from build123d import *

# Parameters (mm, degrees)
F1_DEPTH  = 15
F2_R      = 3.5
F3_DEPTH  = 25
F5_D      = 6.6
F5_DEPTH  = 15
F5_TIP    = 1.9828400428
F6_SIZE   = 10
F7_W      = 6.5
F7_H      = 6.5
F8_DEPTH  = 12.8004791855
F10_D     = 4.4
F10_DEPTH = 5
F10_TIP   = 1.3218933619
F11_SIZE  = 0.25
F12_R     = 0.25


with BuildPart() as f1:
    # F0 (on Top) → F1 (new body)
    with BuildSketch(Plane.XY):
        with BuildLine():
            Line((20, -20), (20, 20))
            Line((20, 20), (-20, 20))
            Line((-20, 20), (-20, 1.5))
            Line((-20, 1.5), (-7.7562877719, 1.5))
            ThreePointArc((-7.7562877719, 1.5), (7.9, 0), (-7.7562877719, -1.5))
            Line((-7.7562877719, -1.5), (-20, -1.5))
            Line((-20, -1.5), (-20, -20))
            Line((-20, -20), (20, -20))
        make_face()
    extrude(amount=F1_DEPTH)

    # F2 (on Front) → F3 (cut)
    with BuildSketch(Plane.XZ):
        with Locations((-14, 7.5)):
            Circle(F2_R)
    extrude(amount=F3_DEPTH, mode=Mode.SUBTRACT)

    # F5
    with Locations(Plane.XZ.offset(-1.5)):
        with Locations((-14, 7.5)):
            Hole(F5_D / 2, depth=F5_DEPTH)
            with Locations((0, 0, -(F5_DEPTH + F5_TIP / 2))):  # 118° drill point
                Cone(0, F5_D / 2, F5_TIP, mode=Mode.SUBTRACT)

    # F6
    f6_edges = [f1.edges().sort_by_distance(p)[0] for p in [
        (20, -20, 7.5),
        (20, 20, 7.5),
    ]]
    chamfer(f6_edges, length=F6_SIZE)

    # F7 (on face) → F8 (cut, through all)
    with BuildSketch(Plane.YZ.offset(20)):
        with Locations((0, 7.5)):
            Rectangle(F7_W, F7_H)
    extrude(amount=-F8_DEPTH, mode=Mode.SUBTRACT)

    # F10
    with Locations(Plane(origin=(0, 0, 0), x_dir=(1, 0, 0), z_dir=(0, 0, -1))):
        with Locations((14, 0)):
            Hole(F10_D / 2, depth=F10_DEPTH)
            with Locations((0, 0, -(F10_DEPTH + F10_TIP / 2))):  # 118° drill point
                Cone(0, F10_D / 2, F10_TIP, mode=Mode.SUBTRACT)

    # F11
    f11_edges = [f1.edges().sort_by_distance(p)[0] for p in [
        (-17.5, -20, 7.5),
        (11.8, 0, 0),
    ]]
    chamfer(f11_edges, length=F11_SIZE)

    # F12
    f12_edges = [f1.edges().sort_by_distance(p)[0] for p in [
        (13.60026, 3.25, 4.25),
        (13.60026, -3.25, 4.25),
        (13.60026, 3.25, 10.75),
        (13.60026, -3.25, 10.75),
    ]]
    fillet(f12_edges, radius=F12_R)


solid = f1.part
Check sheet for the modelled part. Datum: model origin and axes. Units: mm. A direction names the side the tool comes from. Round coordinates to 2 decimals unless told otherwise and drop trailing zeros. Loops run counter-clockwise (first coordinate to the right, second up) from the corner with the lowest first, then second, coordinate; pieces in that order, holes last.
1. Gauge pin test, flat ends, axial feed: pin 1 Ø3.5 at (x, y) = (14, 0) entering from -Z; pin 2 Ø6.5 at (x, z) = (15, 6.5) entering from +Y; pin 3 Ø5.5 at (x, z) = (-14, 7.5) entering from -Y. Record the tip position at first contact, or that the pin passes through.
2. Scan lines: probe 1 along Y at (x, z) = (8, 9.5); probe 2 along X at (y, z) = (0, 2.9); probe 3 along Y at (x, z) = (0, 8.75). Record each from-to range of solid material in increasing order.
3. Sectioned sample at A-A on y = 0. Record the boundary of the cut face in (x, z), and give its area (3 significant figures).
4. Sectioned sample at D-D on y = 6. Record the boundary of the cut face in (x, z), and give its area (3 significant figures).
5. Set-up check for faces 1 (the flat face through (14, 0, 10.75)), 2 (the cylindrical face through (-11.381, 9.105, 5.492)), 3 (the cylindrical face through (11.968, 0.843, 2.278)), 4 (the flat face through (-14, 1.5, 4)): record each of +Z, -Z, +X, -X, +Y, -Y from which the full face is reachable in a straight line by a thin tool's end or side.
6. Sectioned sample at C-C on z = 1.75. Record the boundary of the cut face in (x, y).
7. Mould release check, pull along Z, two halves, no side actions. Record for faces 5 (the flat face through (-12, -1.5, 4)), 6 (the cylindrical face through (-10.767, -10.497, 6.159)), 7 (the flat face through (-9, -4, 0)): released by +Z, released by -Z, zero draft, split by the parting line, or undercut.
8. Sectioned sample at B-B on x = -9. Record the boundary of the cut face in (y, z), and give its area (3 significant figures).
Recorded:
1. pin 1: stops at z = 10.75
1. pin 2: stops at y = 18.25
1. pin 3: stops at y = 16.83
2. probe 1: y = -20 to -3.25, 3.25 to 20
2. probe 2: x = 7.9 to 11.8, 16.2 to 20
2. probe 3: y = -20 to -7.9, 7.9 to 20
3. outline: (7.9, 0) - (11.55, 0) - (11.8, 0.25) - (11.8, 4.25) - (7.9, 4.25) - close; (7.9, 10.75) - (20, 10.75) - (20, 15) - (7.9, 15) - close; (16.2, 0.25) - (16.45, 0) - (20, 0) - (20, 4.25) - (16.2, 4.25) - close
3. area: 84.1 mm2
4. outline: (-20, 0) - (-5.14, 0) - (-5.14, 15) - (-20, 15) - close; (5.14, 0) - (20, 0) - (20, 15) - (5.14, 15) - close; hole circle Ø6.6 at (-14, 7.5)
4. area: 412 mm2
5. face 1: +X
5. face 2: -Y
5. face 3: -Z
5. face 4: +Z, -Z, -X
6. outline: (-20, -20) - (10, -20) - (20, -10) - (20, 10) - (10, 20) - (-20, 20) - (-20, 1.5) - (-7.76, 1.5) arc R7.9 cw (long way) to (-7.76, -1.5) - (-20, -1.5) - close; hole circle Ø4.4 at (14, 0)
7. face 5: zero draft
7. face 6: undercut
7. face 7: released by -Z
8. outline: (-20, 0) - (-1.5, 0) - (-1.5, 15) - (-20, 15) - close; (1.5, 0) - (20, 0) - (20, 15) - (1.5, 15) - close
8. area: 555 mm2
